The listing builds one solid part. Answer for the finished solid, in the listing's coordinates (mm). A direction names the side the tool comes from. Coordinates: 2 decimals unless noted, no trailing zeros. Loops run counter-clockwise (first coordinate to the right, second up) from the corner with the lowest first, then second, coordinate; pieces in that order, holes last. Notation, with made-up numbers: (0.25, -16.75) -> (36.25, -16.75) arc R8 ccw to (36.25, -8.75) -> close; hole circle Ø6 at (23.5, 5.5). An arc over 180 degrees is marked (long way). Answer in a Markdown table with one row per item.
```python
from build123d import *

# Parameters (mm, degrees)
EXTRUDE_1_DEPTH   = 21
EXTRUDE_1_2_DEPTH = 2.2


with BuildPart() as part:
    # 草图2 → Extrude 1 (new body)
    with BuildSketch(Plane(origin=(0, 0, 0), x_dir=(1, 0, 0), z_dir=(0, 1, 0))):
        with BuildLine():
            Line((-11.5, -5.75), (-11.5, -16.75))
            ThreePointArc((-11.5, -16.75), (-10.621320344, -18.871320344), (-8.5, -19.75))
            Line((-8.5, -19.75), (8.5, -19.75))
            ThreePointArc((8.5, -19.75), (10.621320344, -18.871320344), (11.5, -16.75))
            Line((11.5, -16.75), (11.5, 16.75))
            ThreePointArc((11.5, 16.75), (10.621320344, 18.871320344), (8.5, 19.75))
            Line((8.5, 19.75), (-8.5, 19.75))
            ThreePointArc((-8.5, 19.75), (-10.621320344, 18.871320344), (-11.5, 16.75))
            Line((-11.5, 16.75), (-11.5, 5.75))
            Line((-11.5, 5.75), (-13, 5.75))
            Line((-13, 5.75), (-13, 16.75))
            ThreePointArc((-13, 16.75), (-11.681980515, 19.931980515), (-8.5, 21.25))
            Line((-8.5, 21.25), (8.5, 21.25))
            ThreePointArc((8.5, 21.25), (11.681980515, 19.931980515), (13, 16.75))
            Line((13, 16.75), (13, -16.75))
            ThreePointArc((13, -16.75), (11.681980515, -19.931980515), (8.5, -21.25))
            Line((8.5, -21.25), (-8.5, -21.25))
            ThreePointArc((-8.5, -21.25), (-11.681980515, -19.931980515), (-13, -16.75))
            Line((-13, -16.75), (-13, -5.75))
            Line((-13, -5.75), (-11.5, -5.75))
        make_face()
    extrude(amount=EXTRUDE_1_DEPTH)

    # 草图3 → Extrude 1 2 (add)
    with BuildSketch(Plane(origin=(0, 0, 0), x_dir=(1, 0, 0), z_dir=(0, 1, 0))):
        with BuildLine():
            Line((-8.5, -19.75), (8.5, -19.75))
            ThreePointArc((8.5, -19.75), (10.621320344, -18.871320344), (11.5, -16.75))
            Line((11.5, -16.75), (11.5, 16.75))
            ThreePointArc((11.5, 16.75), (10.621320344, 18.871320344), (8.5, 19.75))
            Line((8.5, 19.75), (-8.5, 19.75))
            ThreePointArc((-8.5, 19.75), (-10.621320344, 18.871320344), (-11.5, 16.75))
            Line((-11.5, 16.75), (-11.5, 5.75))
            Line((-11.5, 5.75), (-11.5, 0))
            Line((-11.5, 0), (-11.5, -5.75))
            Line((-11.5, -5.75), (-11.5, -16.75))
            ThreePointArc((-11.5, -16.75), (-10.621320344, -18.871320344), (-8.5, -19.75))
        make_face()
    extrude(amount=EXTRUDE_1_2_DEPTH)


solid = part.part
```
Item 1: A cutting plane is placed at B-B, the plane y = 11. Determine the outline of the cut face in (x, z).
Findings below:
| item | result |
|---|---|
| outline | (-13, -16.75) arc R4.5 ccw to (-8.5, -21.25) -> (8.5, -21.25) arc R4.5 ccw to (13, -16.75) -> (13, 16.75) arc R4.5 ccw to (8.5, 21.25) -> (-8.5, 21.25) arc R4.5 ccw to (-13, 16.75) -> (-13, 5.75) -> (-11.5, 5.75) -> (-11.5, 16.75) arc R3 cw to (-8.5, 19.75) -> (8.5, 19.75) arc R3 cw to (11.5, 16.75) -> (11.5, -16.75) arc R3 cw to (8.5, -19.75) -> (-8.5, -19.75) arc R3 cw to (-11.5, -16.75) -> (-11.5, -5.75) -> (-13, -5.75) -> close |
Item 2: A cutting plane is placed at C-C, the plane x = 0.25. Determine the outline of the cut face in (y, z).
Findings below:
| item | result |
|---|---|
| outline | (0, -21.25) -> (21, -21.25) -> (21, -19.75) -> (2.2, -19.75) -> (2.2, 19.75) -> (21, 19.75) -> (21, 21.25) -> (0, 21.25) -> close |
Item 3: A cutting plane is placed at D-D, the plane z = -3. Determine the outline of the cut face in (x, y).
Findings below:
| item | result |
|---|---|
| outline | (-11.5, 0) -> (13, 0) -> (13, 21) -> (11.5, 21) -> (11.5, 2.2) -> (-11.5, 2.2) -> close |
Item 4: Determine the mould class of faces 1 (the face through (0, 11, -19.75)), 2 (the face through (-11.647, 10.353, 19.967)), 3 (the face through (-13, 10, 11)), 4 (the face through (-12, 10, 5.75)) for opening direction Z: +Z half, -Z half, draft (parallel to the pull), parting line (faces both ways), or undercut.
Findings below:
| item | result |
|---|---|
| face 1 | undercut |
| face 2 | +Z half |
| face 3 | draft |
| face 4 | undercut |
Item 5: A cutting plane is placed at A-A, the plane z = 6.5. Determine the outline of the cut face in (x, y).
Findings below:
| item | result |
|---|---|
| outline | (-13, 0) -> (13, 0) -> (13, 21) -> (11.5, 21) -> (11.5, 2.2) -> (-11.5, 2.2) -> (-11.5, 21) -> (-13, 21) -> close |
Item 6: Find the intervals of material crossed by probe 1 along X at (y, z) = (13.25, 7); probe 2 along Z at (x, y) = (4.25, 10.5); probe 3 along Y at (x, z) = (9.75, 2.5), in increasing order.
Findings below:
| item | result |
|---|---|
| probe 1 | x = -13 to -11.5, 11.5 to 13 |
| probe 2 | z = -21.25 to -19.75, 19.75 to 21.25 |
| probe 3 | y = 0 to 2.2 |
Item 7: Flat-ended cylindrical pins translate along their axes: pin 1 Ø1.8 at (y, z) = (1, -2) entering from -X; pin 2 Ø0.8 at (x, y) = (-12.5, 13.5) entering from +Z; pin 3 Ø6 at (x, z) = (1.5, -9) entering from +Y. Find the tip coordinate at first contact, or state that the pin passes through.
Findings below:
| item | result |
|---|---|
| pin 1 | stops at x = -11.5 |
| pin 2 | stops at z = 19.45 |
| pin 3 | stops at y = 2.2 |
Item 8: A tool of negligible diameter and unlimited length cuts with its end or side. For faces 5 (the face through (-11.5, 1, 0)), 6 (the face through (10.64, 11.47, -18.85)), 7 (the face through (0, 10, -21.25)), from which of +Z, -Z, +X, -X, +Y, -Y can it reach the whole face along a straight path? Write none if from no direction.
Findings below:
| item | result |
|---|---|
| face 5 | -X, +Y, -Y |
| face 6 | +Y |
| face 7 | -Z, +X, -X, +Y, -Y |
